from build123d import *

# Parameters (mm, degrees)
F0_R     = 19.05
F1_DEPTH = 2.54
F3_DEPTH = 6.35


with BuildPart() as f1:
    # F0 (on Top) → F1 (new body)
    with BuildSketch(Plane.XY):
        Circle(F0_R)
    extrude(amount=F1_DEPTH)

    # F2 (on face) → F3 (join)
    with BuildSketch(Plane.XY.offset(2.54)):
        with BuildLine():
            Line((15.824118, -1.27), (-15.824118, -1.27))
            ThreePointArc((-15.824118, -1.27), (0, -15.875), (15.824118, -1.27))
        make_face()
        with BuildLine():
            Line((-15.824118, 1.27), (15.824118, 1.27))
            ThreePointArc((15.824118, 1.27), (0, 15.875), (-15.824118, 1.27))
        make_face()
    extrude(amount=F3_DEPTH)


solid = f1.part
Check sheet for the modelled part. Datum: model origin and axes. Units: mm. A direction names the side the tool comes from. Round coordinates to 2 decimals unless told otherwise and drop trailing zeros. Order: outer loops, then holes, each group sorted by start corner. A loop starts at its lowest first (then second) coordinate and runs counter-clockwise, first axis right, second up.
(1) Cross-section at A-A, the plane z = 5.75. Enter the section's corners in (x, y) (3 decimals), and give its area (3 significant figures).
(2) Draft check along Y on faces 4 (the flat face through (0, 7, 8.89)), 5 (the flat face through (0, -1.27, 6)), 6 (the cylindrical face through (-15.12, -11.59, 1.25)). Enter one of: pulls with the +Y half, pulls with the -Y half, needs draft (parallel to the pull), parting line crosses it, or undercut.
(3) Cross-section at C-C, the plane y = -3. Enter the section's corners in (x, z), and give its area (3 significant figures).
(4) Scan lines: probe 1 along Y at (x, z) = (-8.5, 4); probe 2 along Y at (x, z) = (5, 7.5); probe 3 along Z at (x, y) = (12, 11). Record each from-to range of solid material in increasing order.
(5) Cross-section at D-D, the plane x = 13. Enter the section's corners in (y, z), and give its area (3 significant figures).
(6) Cross-section at B-B, the plane x = 0. Enter the section's corners in (y, z) (3 decimals).
(7) Access from +Z, -Z, +X, -X, +Y, -Y to the whole of each face (thin tool, end or side, straight path). Record for faces 1 (the flat face through (0, 1.27, 6)), 2 (the cylindrical face through (-0.33, -15.87, 5.67)), 3 (the cylindrical face through (0.33, 15.87, 5.67)).
(8) Go/stop test with flat-tipped pins: P1, Ø5, axis at x = 14, z = 6.5, coming from the +Y side; P2, Ø3, axis at x = 10, z = 4.5, coming from the -Y side; P3, Ø3, axis at x = -1, z = 5.5, coming from the +Y side (3 decimals). Record where each tip stops, or that it passes through.
Check sheet entries:
1. outline: (-15.824, -1.27) arc R15.875 ccw to (15.824, -1.27) - close; (-15.824, 1.27) - (15.824, 1.27) arc R15.875 ccw to start
1. area: 711 mm2
2. face 4: needs draft
2. face 5: undercut
2. face 6: parting line crosses it
3. outline: (-18.81, 0) - (18.81, 0) - (18.81, 2.54) - (15.59, 2.54) - (15.59, 8.89) - (-15.59, 8.89) - (-15.59, 2.54) - (-18.81, 2.54) - close
3. area: 294 mm2
4. probe 1: y = -13.41 to -1.27, 1.27 to 13.41
4. probe 2: y = -15.07 to -1.27, 1.27 to 15.07
4. probe 3: z = 0 to 2.54
5. outline: (-13.92, 0) - (13.92, 0) - (13.92, 2.54) - (9.11, 2.54) - (9.11, 8.89) - (1.27, 8.89) - (1.27, 2.54) - (-1.27, 2.54) - (-1.27, 8.89) - (-9.11, 8.89) - (-9.11, 2.54) - (-13.92, 2.54) - close
5. area: 170 mm2
6. outline: (-19.05, 0) - (19.05, 0) - (19.05, 2.54) - (15.875, 2.54) - (15.875, 8.89) - (1.27, 8.89) - (1.27, 2.54) - (-1.27, 2.54) - (-1.27, 8.89) - (-15.875, 8.89) - (-15.875, 2.54) - (-19.05, 2.54) - close
7. face 1: +Z, +X, -X
7. face 2: +Z, -Y
7. face 3: +Z, +Y
8. P1: stops at y = 10.94
8. P2: stops at y = -13.41
8. P3: stops at y = 15.875
